Can you work these out from the drawing? Everything is in mm from the part's minimum corner. Round coordinates to 2 decimals unless told otherwise and drop trailing zeros. Order: outer loops, then holes, each group sorted by start corner. A loop starts at its lowest first (then second) coordinate and runs counter-clockwise, first axis right, second up. Notation, with made-up numbers: (51, 71) - (83, 71) arc R17 ccw to (83, 99) - close; hole circle Ø10 at (-21.75, -31). An arc over 180 degrees is marked (long way). Answer as a JSON object with one key per item and string values.
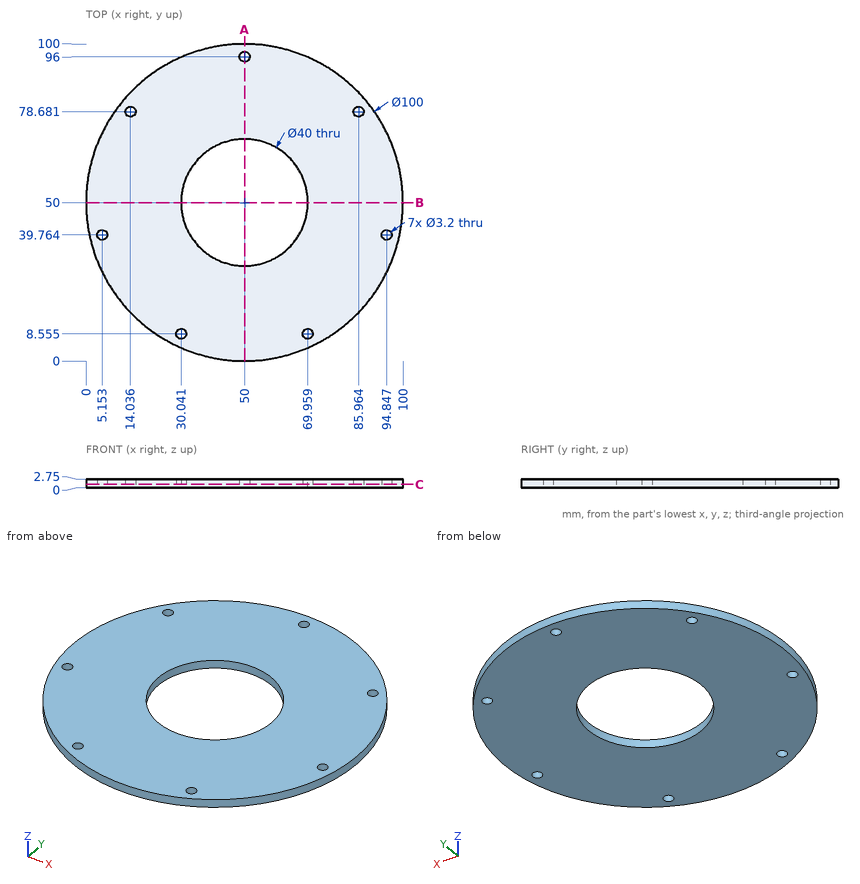
1. Imagine slicing it at B-B (y = 50). List the corners of the cut face in (x, z) for me, plus the area to 3 significant figures.
Responses:
{"outline": "(0, 0) - (30, 0) - (30, 2.75) - (0, 2.75) - close; (70, 0) - (100, 0) - (100, 2.75) - (70, 2.75) - close", "area": "165 mm2"}
2. Imagine slicing it at A-A (x = 50). List the corners of the cut face in (y, z) for me, plus the area to 3 significant figures.
Responses:
{"outline": "(0, 0) - (30, 0) - (30, 2.75) - (0, 2.75) - close; (70, 0) - (94.4, 0) - (94.4, 2.75) - (70, 2.75) - close; (97.6, 0) - (100, 0) - (100, 2.75) - (97.6, 2.75) - close", "area": "156 mm2"}
3. If I drill on L1, parallel to X at y = 83, z = 0.35 (1 decimal); L2, parallel to X at y = 59.5, z = 1.6; L3, parallel to Y at x = 48, z = 0.8, over which ranges is the centre line in solid material (lowest first)? Write a range as [from, to].
Responses:
{"L1": "[12.4, 87.6]", "L2": "[0.91, 32.4], [67.6, 99.09]", "L3": "[0.04, 30.1], [69.9, 99.96]"}
4. Imagine slicing it at C-C (z = 1.05). Give the number of separate pieces and of enclosed holes in the cut face, plus the area to 3 significant figures.
Responses:
{"separate pieces": "1", "enclosed holes": "8", "area": "6,540 mm2"}
5. For P1, Ø3, axis at x = 5.15, y = 39.76, coming from the +Z side, with a flat end and sliding along its axis, tell me the tip position at first contact or that it passes through.
Responses:
{"P1": "through"}
